Geometry check sheet. Reference: the model listing, model coordinates, mm. A direction names the side the tool comes from. Round coordinates to 2 decimals unless told otherwise and drop trailing zeros. Write each loop counter-clockwise with the first axis right and the second up, starting at its lowest first coordinate (ties: lowest second). Pieces come first, ordered by that corner, then holes. Notation, with made-up numbers: (44.25, 79.25) - (102.25, 79.25) arc R22 cw to (102.25, 105.25) - close; hole circle Ø3 at (7, -40). An arc over 180 degrees is marked (long way). Return JSON: item names as keys, results as strings. Group by question number.
from build123d import *

# Parameters (mm, degrees)
SKETCH4_W            = 69.2
SKETCH4_H            = 45.8
SKETCH4_W_2          = 30
SKETCH4_H_2          = 30
BOSS_EXTRUDE11_DEPTH = 10
SKETCH9_W            = 69.2
SKETCH9_H            = 45.8
BOSS_EXTRUDE12_DEPTH = 10
SKETCH10_W           = 15
SKETCH10_H           = 45.8
BOSS_EXTRUDE13_DEPTH = 100
MOVE_FACE2_BY        = 4.7
MOVE_FACE3_BY        = 10
SKETCH11_W           = 25
SKETCH11_H           = 25
CUT_EXTRUDE1_DEPTH   = 10
MOVE_FACE4_BY        = 10


with BuildPart() as part:
    # Sketch4 → Boss-Extrude11 (new body)
    with BuildSketch(Plane(origin=(0, 0, 0), x_dir=(1, 0, 0), z_dir=(0, 1, 0))):
        Rectangle(SKETCH4_W, SKETCH4_H)
        Rectangle(SKETCH4_W_2, SKETCH4_H_2, mode=Mode.SUBTRACT)
    extrude(amount=BOSS_EXTRUDE11_DEPTH)

    # Sketch9 → Boss-Extrude12 (add)
    with BuildSketch(Plane(origin=(0, 10, 0), x_dir=(1, 0, 0), z_dir=(0, 1, 0))):
        Rectangle(SKETCH9_W, SKETCH9_H)
    extrude(amount=BOSS_EXTRUDE12_DEPTH)

    # Sketch10 → Boss-Extrude13 (add)
    with BuildSketch(Plane(origin=(0, 20, 0), x_dir=(1, 0, 0), z_dir=(0, 1, 0))):
        with Locations((27.1, 0)):
            Rectangle(SKETCH10_W, SKETCH10_H)
    extrude(amount=BOSS_EXTRUDE13_DEPTH)

    # Move Face2: a face moved inward by 4.7
    extrude(part.faces().sort_by_distance((0, 12, -22.9))[0], amount=MOVE_FACE2_BY, dir=(0, 0, 1), mode=Mode.SUBTRACT)

    # Move Face3: a face moved outward by 10.0
    extrude(part.faces().sort_by_distance((0, 10, 0))[0], amount=MOVE_FACE3_BY, dir=(0, -1, 0))

    # Sketch11 → Cut-Extrude1 (cut)
    with BuildSketch(Plane.XZ):
        with Locations((-4.99, 7.35)):
            Rectangle(SKETCH11_W, SKETCH11_H)
    extrude(amount=-CUT_EXTRUDE1_DEPTH, mode=Mode.SUBTRACT)

    # Move Face4: a face moved inward by 10.0
    extrude(part.faces().sort_by_distance((27.1, 120, 2.35))[0], amount=MOVE_FACE4_BY, dir=(0, -1, 0), mode=Mode.SUBTRACT)


solid = part.part
1. Material ranges on line 1 along X through (y, z) = (80.5, -1.5); line 2 along Y through (x, z) = (-19, 0); line 3 along X through (y, z) = (6, 16), recorded low to high.
2. Section check C-C (y = 73). Enter the section's corners in (x, z), and give its area (4 significant figures).
3. Depth check by flat-ended pin: pin 1 Ø12 at (y, z) = (86, 18) entering from -X; pin 2 Ø3 at (x, z) = (3, 15) entering from +Y. Enter the tip coordinate at first touch or a pass-through.
4. Section check A-A (x = -8). Enter the section's corners in (y, z), and give its area (3 significant figures).
5. Section check B-B (z = 15). Enter the section's corners in (x, y).
6. Tool access check on faces 1 (the face through (-8, 20, 2)), 2 (the face through (-5, 5, -5.15)), 3 (the face through (27, 110, 2)). Record the directions out of +Z, -Z, +X, -X, +Y, -Y that give a thin tool (end or side, any length) a straight path to the whole face; none if there is none.
7. Section check D-D (z = -14). Enter the section's corners in (x, y).
8. Mould release check, pull along X, two halves, no side actions. Record for faces 4 (the face through (-34.6, 10, 3)), 5 (the face through (-5, 5, 19.85)), 6 (the face through (-17.49, 5, 7)), 7 (the face through (23, 30, 22.9)): pulls with the +X half, pulls with the -X half, needs draft (parallel to the pull), parting line crosses it, or undercut.
Result sheet:
{
 "1": {"line 1": "x = 19.6 to 34.6", "line 2": "y = 0 to 20", "line 3": "x = -34.6 to -17.49, 7.51 to 34.6"},
 "2": {"outline": "(19.6, -18.2) - (34.6, -18.2) - (34.6, 22.9) - (19.6, 22.9) - close", "area": "616.5 mm²"},
 "3": {"pin 1": "stops at x = 19.6", "pin 2": "stops at y = 20"},
 "4": {"outline": "(0, -18.2) - (20, -18.2) - (20, 22.9) - (0, 22.9) - (0, 19.85) - (10, 19.85) - (10, -5.15) - (0, -5.15) - close", "area": "572 mm²"},
 "5": {"outline": "(-34.6, 0) - (-17.49, 0) - (-17.49, 10) - (7.51, 10) - (7.51, 0) - (34.6, 0) - (34.6, 110) - (19.6, 110) - (19.6, 20) - (-34.6, 20) - close"},
 "6": {"face 1": "+Z, -Z, -X, +Y", "face 2": "-Y", "face 3": "+Z, -Z, +X, -X, +Y"},
 "7": {"outline": "(-34.6, 0) - (34.6, 0) - (34.6, 110) - (19.6, 110) - (19.6, 20) - (-34.6, 20) - close"},
 "8": {"face 4": "pulls with the -X half", "face 5": "undercut", "face 6": "undercut", "face 7": "needs draft"}
}
